Check sheet for the modelled part. Datum: model origin and axes. Units: mm. A direction names the side the tool comes from. Round coordinates to 2 decimals unless told otherwise and drop trailing zeros. Loops run counter-clockwise (first coordinate to the right, second up) from the corner with the lowest first, then second, coordinate; pieces in that order, holes last. Notation, with made-up numbers: M 40.25,-6.75 L 94.25,-6.75 A13 ccw 94.25,-2.75 Z; hole C -6,-30 d4. An arc over 180 degrees is marked long. Write item = value, one per line. Start each with the question number.
(1) Scan lines: L1, parallel to Y at x = 242, z = 0; L2, parallel to Y at x = 19, z = 0; L3, parallel to X at y = -6, z = 2.75. Record each from-to range of solid material in increasing order. Write a range as from..to.
(2) Cross-section at A-A on x = 178. Record the boundary of the cut face in (y, z).
(3) Go/stop test with flat-tipped pins: P1, Ø5.5, axis at y = 0, z = 0, coming from the +X side; P2, Ø6, axis at x = 45.5, y = 7.5, coming from the +Z side; P3, Ø5, axis at x = 97.5, z = 5.5, coming from the -Y side. Record where each tip stops, or that it passes through.
(4) Mould release check, pull along Z, two halves, no side actions. Record for faces 1 (the face through (52.51, -7.84, 5)), 2 (the face through (39.61, -0.72, -0.16)), 3 (the face through (53.2, 9, -3)): pulls with the +Z half, pulls with the -Z half, needs draft (parallel to the pull), parting line crosses it, or undercut.
(5) Set-up check for faces 4 (the face through (19.629, 3.584, -2.285)), 5 (the face through (245.06, 7.81, -1.73)), 6 (the face through (240.5, -7, 0)): record each of +Z, -Z, +X, -X, +Y, -Y from which the full face is reachable in a straight line by a thin tool's end or side.
from build123d import *

# Parameters (mm, degrees)
M10X1_52_D            = 8.5
M10X1_52_DEPTH        = 37.5
M10X1_52_CSINK_D      = 11
M10X1_52_CSINK_ANGLE  = 90
M10X1_52_TIP          = 2.553657631
HOLE_WIZARD_M81_D     = 6.8
HOLE_WIZARD_M81_DEPTH = 20
HOLE_WIZARD_M81_TIP   = 2.042926105
SKETCH_6_W            = 2
SKETCH_6_H            = 1.5
SKETCH_20_W           = 1.4
SKETCH_20_H           = 0.7
CHAMFER_1_SIZE        = 1


with BuildPart() as part:
    # Эскиз1 → Повернуть1 (revolve)
    with BuildSketch(Plane.XY, mode=Mode.PRIVATE) as revolve_1_sk:
        Polygon((0, 10), (238.5, 10), (238.5, 8), (250.5, 8), (250.5, 0), (0, 0), align=None)
    revolve(revolve_1_sk.sketch.rotate(Axis((-123.335902371, 0, 0), (1, 0, 0)), 90), axis=Axis((-123.335902371, 0, 0), (1, 0, 0)))

    # Отверстие обработанное метчиком M10x1.52
    with Locations(Plane.ZY):
        with Locations((0, 0)):
            CounterSinkHole(M10X1_52_D / 2, M10X1_52_CSINK_D / 2, depth=M10X1_52_DEPTH, counter_sink_angle=M10X1_52_CSINK_ANGLE)
            with Locations((0, 0, -(M10X1_52_DEPTH + M10X1_52_TIP / 2))):  # 118° drill point
                Cone(0, M10X1_52_D / 2, M10X1_52_TIP, mode=Mode.SUBTRACT)

    # Отверстие обработанное метчиком M81
    with Locations(Plane(origin=(250.5, 0, 0), x_dir=(0, 0, -1), z_dir=(1, 0, 0))):
        with Locations((0, 0)):
            Hole(HOLE_WIZARD_M81_D / 2, depth=HOLE_WIZARD_M81_DEPTH)
            with Locations((0, 0, -(HOLE_WIZARD_M81_DEPTH + HOLE_WIZARD_M81_TIP / 2))):  # 118° drill point
                Cone(0, HOLE_WIZARD_M81_D / 2, HOLE_WIZARD_M81_TIP, mode=Mode.SUBTRACT)

    # Эскиз6 → Вырез-Повернуть1 (revolve, cut)
    with BuildSketch(Plane.XY, mode=Mode.PRIVATE) as cut_revolve_1_sk:
        with Locations((239.5, 7.25)):
            Rectangle(SKETCH_6_W, SKETCH_6_H)
    revolve(cut_revolve_1_sk.sketch.rotate(Axis((0, 0, 0), (1, 0, 0)), 90), axis=Axis((0, 0, 0), (1, 0, 0)), mode=Mode.SUBTRACT)

    # Эскиз20 → Вырез-Повернуть2 (revolve, cut)
    with BuildSketch(Plane.XY, mode=Mode.PRIVATE) as cut_revolve_2_sk:
        with Locations((52.5, 9.65)):
            Rectangle(SKETCH_20_W, SKETCH_20_H)
    revolve(cut_revolve_2_sk.sketch.rotate(Axis((0, 0, 0), (1, 0, 0)), 90), axis=Axis((0, 0, 0), (1, 0, 0)), mode=Mode.SUBTRACT)

    # Фаска1
    chamfer_1_edges = [part.edges().sort_by_distance(p)[0] for p in [
        (250.5, 0, -8),
        (0, 0, -10),
    ]]
    chamfer(chamfer_1_edges, length=CHAMFER_1_SIZE)


solid = part.part
Result:
q1.L1 = -8..-3.4, 3.4..8
q1.L2 = -10..-4.25, 4.25..10
q1.L3 = 0..238.5, 240.5..250.5
q2.outline = C 0,0 d20
q3.P1 = 230.11
q3.P2 = 8.93
q3.P3 = -9.54
q4.face_1 = parting line crosses it
q4.face_2 = undercut
q4.face_3 = needs draft
q5.face_4 = -X
q5.face_5 = +X
q5.face_6 = none
